```python
from build123d import *

# Parameters (mm, degrees)
F0_R     = 2
F0_R_2   = 1.5
F0_R_3   = 7.5
F1_DEPTH = 2.5


# Not quite as in the source:
# - ends of sketch curves that miss each other by under 0.0002 mm in the source are joined


with BuildPart() as f1:
    # F0 (on Top) → F1 (new body)
    with BuildSketch(Plane.XY):
        with BuildLine():
            Line((-115.919333, 58.73247), (-148.25, 24.5))
            Line((-148.25, 24.5), (-148.25, -24.5))
            Line((-148.25, -24.5), (-115.919333, -58.732471))
            ThreePointArc((-115.919333, -58.732471), (-109.2958427864, -63.3664016249), (-101.37907, -65))
            Line((-101.37907, -65), (-17.75, -65))
            Line((-17.75, -65), (145.974987, -50.205574))
            ThreePointArc((145.974987, -50.205574), (147.5955984677, -49.4020650272), (148.25, -47.715718))
            Line((148.25, -47.715718), (148.25, -36.5))
            Line((148.25, -36.5), (148.25, 47.715717))
            ThreePointArc((148.25, 47.715717), (147.5955984677, 49.4020640272), (145.9749869631, 50.2055725915))
            Line((145.9749869631, 50.2055725915), (-17.75, 65))
            Line((-17.75, 65), (-101.37907, 65))
            ThreePointArc((-101.37907, 65), (-109.2958431202, 63.366401481), (-115.919333, 58.73247))
        make_face()
        with Locations((-112.25, -40)):
            Circle(F0_R, mode=Mode.SUBTRACT)
        with BuildLine():
            ThreePointArc((-49.75, -63), (-52.2248737342, -61.9748737342), (-53.25, -59.5))
            ThreePointArc((-53.25, -59.5), (-52.2248737342, -57.0251262658), (-49.75, -56))
            Line((-49.75, -56), (-39.75, -56))
            ThreePointArc((-39.75, -56), (-37.2751262658, -57.0251262658), (-36.25, -59.5))
            ThreePointArc((-36.25, -59.5), (-37.2751262658, -61.9748737342), (-39.75, -63))
            Line((-39.75, -63), (-49.75, -63))
        make_face(mode=Mode.SUBTRACT)
        with Locations((-71, -43)):
            Circle(F0_R_2, mode=Mode.SUBTRACT)
        with Locations((-12.75, -45)):
            Circle(F0_R_2, mode=Mode.SUBTRACT)
        with Locations((-138.25, -12)):
            Circle(F0_R_2, mode=Mode.SUBTRACT)
        with Locations((-128.25, -12)):
            Circle(F0_R_2, mode=Mode.SUBTRACT)
        with BuildLine():
            ThreePointArc((-23.25, -27.5), (-25.017766953, -26.767766953), (-25.75, -25))
            ThreePointArc((-25.75, -25), (-25.017766953, -23.232233047), (-23.25, -22.5))
            Line((-23.25, -22.5), (-13.75, -22.5))
            ThreePointArc((-13.75, -22.5), (-11.982233047, -23.232233047), (-11.25, -25))
            ThreePointArc((-11.25, -25), (-11.982233047, -26.767766953), (-13.75, -27.5))
            Line((-13.75, -27.5), (-23.25, -27.5))
        make_face(mode=Mode.SUBTRACT)
        with Locations((20.5, -51.5)):
            Circle(F0_R_2, mode=Mode.SUBTRACT)
        with Locations((38.5, -51.5)):
            Circle(F0_R_2, mode=Mode.SUBTRACT)
        with Locations((67.75, -45)):
            Circle(F0_R_2, mode=Mode.SUBTRACT)
        with Locations((91.75, -44)):
            Circle(F0_R, mode=Mode.SUBTRACT)
        with Locations((134, -40)):
            Circle(F0_R, mode=Mode.SUBTRACT)
        with BuildLine():
            ThreePointArc((12.75, -27.5), (10.982233047, -26.767766953), (10.25, -25))
            ThreePointArc((10.25, -25), (10.982233047, -23.232233047), (12.75, -22.5))
            Line((12.75, -22.5), (22.25, -22.5))
            ThreePointArc((22.25, -22.5), (24.017766953, -23.232233047), (24.75, -25))
            ThreePointArc((24.75, -25), (24.017766953, -26.767766953), (22.25, -27.5))
            Line((22.25, -27.5), (12.75, -27.5))
        make_face(mode=Mode.SUBTRACT)
        with Locations((58.75, -16)):
            Circle(F0_R_2, mode=Mode.SUBTRACT)
        with Locations((97.75, -16)):
            Circle(F0_R_2, mode=Mode.SUBTRACT)
        with Locations((-138.25, 12)):
            Circle(F0_R_2, mode=Mode.SUBTRACT)
        with Locations((-128.25, 12)):
            Circle(F0_R_2, mode=Mode.SUBTRACT)
        with BuildLine():
            ThreePointArc((-106.6046121633, 25.7917838577), (-105.7465725985, 28.7775878211), (-104.2499995126, 31.4999996564))
            Line((-104.2499995126, 31.4999996564), (-99.481118, 39.303625))
            Line((-99.481118, 39.303625), (-97.347914, 40.5))
            Line((-97.347914, 40.5), (-87.75, 40.5))
            Line((-87.75, 40.5), (-85.25, 38))
            Line((-85.25, 38), (-82.75, 35.5))
            Line((-82.75, 35.5), (-34, 35.5))
            Line((-34, 35.5), (-28, 29.5))
            Line((-28, 29.5), (-28, 24))
            Line((-28, 24), (-23, 19))
            Line((-23, 19), (5.25, 19))
            Line((5.25, 19), (24, 0.25))
            Line((24, 0.25), (24, -0.25))
            Line((24, -0.25), (5.25, -19))
            Line((5.25, -19), (-23, -19))
            Line((-23, -19), (-28, -24))
            Line((-28, -24), (-28, -30))
            Line((-28, -30), (-25, -33))
            Line((-25, -33), (-24.25, -33))
            Line((-24.25, -33), (-20.75, -36.5))
            Line((-20.75, -36.5), (-24.25, -40))
            Line((-24.25, -40), (-70.75, -40))
            Line((-70.75, -40), (-73, -39))
            Line((-73, -39), (-96.75, -39))
            ThreePointArc((-96.75, -39), (-102.9744154707, -36.7847551324), (-106.3997748707, -31.1351909734))
            ThreePointArc((-106.3997748707, -31.1351909734), (-107.7934268918, -2.6763496917), (-106.6046121633, 25.7917838577))
        make_face(mode=Mode.SUBTRACT)
        with BuildLine():
            ThreePointArc((-23.25, 22.5), (-25.017766953, 23.232233047), (-25.75, 25))
            ThreePointArc((-25.75, 25), (-25.017766953, 26.767766953), (-23.25, 27.5))
            Line((-23.25, 27.5), (-13.75, 27.5))
            ThreePointArc((-13.75, 27.5), (-11.982233047, 26.767766953), (-11.25, 25))
            ThreePointArc((-11.25, 25), (-11.982233047, 23.232233047), (-13.75, 22.5))
            Line((-13.75, 22.5), (-23.25, 22.5))
        make_face(mode=Mode.SUBTRACT)
        with Locations((-112.25, 40)):
            Circle(F0_R, mode=Mode.SUBTRACT)
        with Locations((-71, 43)):
            Circle(F0_R_2, mode=Mode.SUBTRACT)
        with Locations((-12.75, 45)):
            Circle(F0_R_2, mode=Mode.SUBTRACT)
        with Locations((58.75, 16)):
            Circle(F0_R_2, mode=Mode.SUBTRACT)
        with BuildLine():
            ThreePointArc((12.75, 22.5), (10.982233047, 23.232233047), (10.25, 25))
            ThreePointArc((10.25, 25), (10.982233047, 26.767766953), (12.75, 27.5))
            Line((12.75, 27.5), (22.25, 27.5))
            ThreePointArc((22.25, 27.5), (24.017766953, 26.767766953), (24.75, 25))
            ThreePointArc((24.75, 25), (24.017766953, 23.232233047), (22.25, 22.5))
            Line((22.25, 22.5), (12.75, 22.5))
        make_face(mode=Mode.SUBTRACT)
        with Locations((75.75, 0)):
            Circle(F0_R_3, mode=Mode.SUBTRACT)
        with Locations((97.75, 16)):
            Circle(F0_R_2, mode=Mode.SUBTRACT)
        with Locations((67.75, 45)):
            Circle(F0_R_2, mode=Mode.SUBTRACT)
        with Locations((91.75, 44)):
            Circle(F0_R, mode=Mode.SUBTRACT)
        with Locations((134, 40)):
            Circle(F0_R, mode=Mode.SUBTRACT)
    extrude(amount=F1_DEPTH)


solid = f1.part
```
Model file for the job. Use its own axes, mm. A direction names the side the tool comes from. Give positions to 0.01 mm unless a question says otherwise; leave off trailing zeros. Write each loop counter-clockwise with the first axis right and the second up, starting at its lowest first coordinate (ties: lowest second). Pieces come first, ordered by that corner, then holes. Notation, with made-up numbers: (75.5, 33) -> (120.5, 33) arc R24 cw to (120.5, 59) -> close; hole circle Ø8 at (53.25, 19). An arc over 180 degrees is marked (long way). Use CSV: the item, a comma, the result in double quotes. Start each with the question number.
1) Cut at B-B on x = 51.5. List the corners of the cut face in (y, z), plus the area to 3 significant figures.
2) Drill centre lines: L1, parallel to Y at x = -58.5, z = 1.45; L2, parallel to Y at x = -112.25, z = 1.55; L3, parallel to Y at x = -129, z = 1.3. Where is each one in solid material? Low to high.
3) Two-plate mould, pull along X, no slides. Class faces 3 (the flat face through (31, 1, 0)), 4 (the cylindrical face through (-109.4, -63.32, 1.23)), 5 (the cylindrical face through (68.257, 0.33, 1.232)), 6 (the flat face through (65.26, 57.5, 1.23)): released by +X, released by -X, zero draft, split by the parting line, or undercut.
4) Cut at A-A on z = 0.95. Count the separate pieces of the cut face and the enclosed holes in it, plus the area to 3 significant figures.
5) Tool access for faces 1 (the flat face through (14.76, -9.49, 1.23)), 2 (the flat face through (31, 1, 2.5)): list every direction of +Z, -Z, +X, -X, +Y, -Y with a clear straight run to the whole face (end or side of a thin tool).
6) Pin check, flat tips, straight feed: P1, Ø2.5, axis at x = 38.5, y = -51.5, coming from the +Z side; P2, Ø1, axis at x = 90.5, z = 0.5, coming from the +Y side. Stop position of each tip, or through.
Final values:
1,outline,"(-58.74, 0) -> (58.74, 0) -> (58.74, 2.5) -> (-58.74, 2.5) -> close"
1,area,"294 mm2"
2,L1,"y = -65 to -40, 35.5 to 65"
2,L2,"y = -61.79 to -42, -38 to 38, 42 to 61.79"
2,L3,"y = -44.88 to -13.3, -10.7 to 10.7, 13.3 to 44.88"
3,face 3,"zero draft"
3,face 4,"released by -X"
3,face 5,"undercut"
3,face 6,"released by +X"
4,separate pieces,"1"
4,enclosed holes,"29"
4,area,"26,100 mm2"
5,face 1,"+Z, -Z"
5,face 2,"+Z, +X, -X, +Y, -Y"
6,P1,"passes through"
6,P2,"stops at y = 55.26"
